```python
from build123d import *

# Parameters (mm, degrees)
F0_W     = 49
F0_H     = 48
F1_DEPTH = 18
F2_W     = 38
F2_H     = 8
F3_DEPTH = 28
F4_W     = 18
F4_H     = 48
F5_DEPTH = 30
F6_W     = 8
F6_H     = 38
F7_DEPTH = 28


with BuildPart() as f1:
    # F0 (on Top) → F1 (new body)
    with BuildSketch(Plane.XY):
        with Locations((-24.5, 24)):
            Rectangle(F0_W, F0_H)
    extrude(amount=F1_DEPTH)

    # F2 (on face) → F3 (cut)
    with BuildSketch(Plane.YZ):
        with Locations((24, 9)):
            Rectangle(F2_W, F2_H)
    extrude(amount=-F3_DEPTH, mode=Mode.SUBTRACT)

    # F4 (on face) → F5 (join)
    with BuildSketch(Plane.XY.offset(18)):
        with Locations((-40, 24)):
            Rectangle(F4_W, F4_H)
    extrude(amount=F5_DEPTH)

    # F6 (on face) → F7 (cut)
    with BuildSketch(Plane.XY.offset(48)):
        with Locations((-40, 24)):
            Rectangle(F6_W, F6_H)
    extrude(amount=-F7_DEPTH, mode=Mode.SUBTRACT)


solid = f1.part
```
Can you work these out from the model? Positions are in its coordinate system, mm. A direction names the side the tool comes from. Give positions to 0.01 mm unless a question says otherwise; leave off trailing zeros. Order: outer loops, then holes, each group sorted by start corner. A loop starts at its lowest first (then second) coordinate and runs counter-clockwise, first axis right, second up. Notation, with made-up numbers: (12.5, -29) - (50.5, -29) arc R27 ccw to (50.5, -12) - close; hole circle Ø11 at (-25.5, -13.75). An arc over 180 degrees is marked (long way). Use a Markdown table: item, result. Add a question column.
Q1. If we section it at D-D on x = -37: Write out the boundary of the cut face in (y, z).
Q2. Please list where these lines run through material, in increasing order: line 1 along X through (y, z) = (7.5, 45); line 2 along Z through (x, y) = (-20, 8.5); line 3 along Y through (x, z) = (-39, 21).
Q3. On a 3-axis mill with a long thin cutter (end or side, diameter ignored), from which of +Z, -Z, +X, -X, +Y, -Y can I reach the whole of each face in a straight line? I mean faces 5 (the flat face through (-16, 24, 18)), 6 (the flat face through (-40, 43, 34)), 7 (the flat face through (-14, 24, 13)). Say none if no direction works.
Q4. I'm going to push flat-ended pins straight in: pin 1 (9 mm diameter, centred on y = 32, z = 32.5, fed in from +X); pin 2 (6.5 mm diameter, centred on x = -40, y = 20.5, fed in from +Z); pin 3 (25 mm diameter, centred on x = -15.5, y = 32.5, fed in from +Z). Where does each tip first touch, or does it pass through?
Q5. If we section it at A-A on x = -17: Write out the boundary of the cut face in (y, z), plus the area to 3 significant figures.
Q6. If we section it at B-B on z = 32.5: Write out the boundary of the cut face in (x, y), plus the area to 3 significant figures.
Q7. If we section it at C-C on y = 8: Write out the boundary of the cut face in (x, z), plus the area to 3 significant figures.
Q8. If we mould it in two halves opening along X, with no side actions, what happens to faces 1 (the flat face through (-25, 24, 0)), 2 (the flat face through (-40, 5, 34)), 3 (the flat face through (-28, 24, 9)), 4 (the flat face through (-36, 24, 34))? For each: released by +X, released by -X, zero draft, split by the parting line, or undercut.
Answers follow:
| question | item | result |
|---|---|---|
| 1 | outline | (0, 0) - (48, 0) - (48, 48) - (43, 48) - (43, 20) - (5, 20) - (5, 48) - (0, 48) - close |
| 2 | line 1 | x = -49 to -44, -36 to -31 |
| 2 | line 2 | z = 0 to 5, 13 to 18 |
| 2 | line 3 | y = 0 to 5, 43 to 48 |
| 3 | face 5 | +Z, +X, +Y, -Y |
| 3 | face 6 | +Z |
| 3 | face 7 | +X |
| 4 | pin 1 | stops at x = -31 |
| 4 | pin 2 | stops at z = 20 |
| 4 | pin 3 | stops at z = 18 |
| 5 | outline | (0, 0) - (48, 0) - (48, 18) - (0, 18) - close; hole (5, 5) - (43, 5) - (43, 13) - (5, 13) - close |
| 5 | area | 560 mm^2 |
| 6 | outline | (-49, 0) - (-31, 0) - (-31, 48) - (-49, 48) - close; hole (-44, 5) - (-36, 5) - (-36, 43) - (-44, 43) - close |
| 6 | area | 560 mm^2 |
| 7 | outline | (-49, 0) - (0, 0) - (0, 5) - (-28, 5) - (-28, 13) - (0, 13) - (0, 18) - (-31, 18) - (-31, 48) - (-36, 48) - (-36, 20) - (-44, 20) - (-44, 48) - (-49, 48) - close |
| 7 | area | 974 mm^2 |
| 8 | face 1 | zero draft |
| 8 | face 2 | undercut |
| 8 | face 3 | released by +X |
| 8 | face 4 | undercut |
